The figure shows three views and two pictorial views of one solid part (mm, origin at its lowest corner). Answer the questions. Give positions to 0.01 mm unless a question says otherwise; leave off trailing zeros. Loops run counter-clockwise (first coordinate to the right, second up) from the corner with the lowest first, then second, coordinate; pieces in that order, holes last. Notation, with made-up numbers: (-20, 83.25) - (15, 83.25) arc R21 cw to (15, 119.25) - close; hole circle Ø1 at (-11, 35). An arc over 180 degrees is marked (long way). Use CSV: the item, a comma, the result in double quotes.
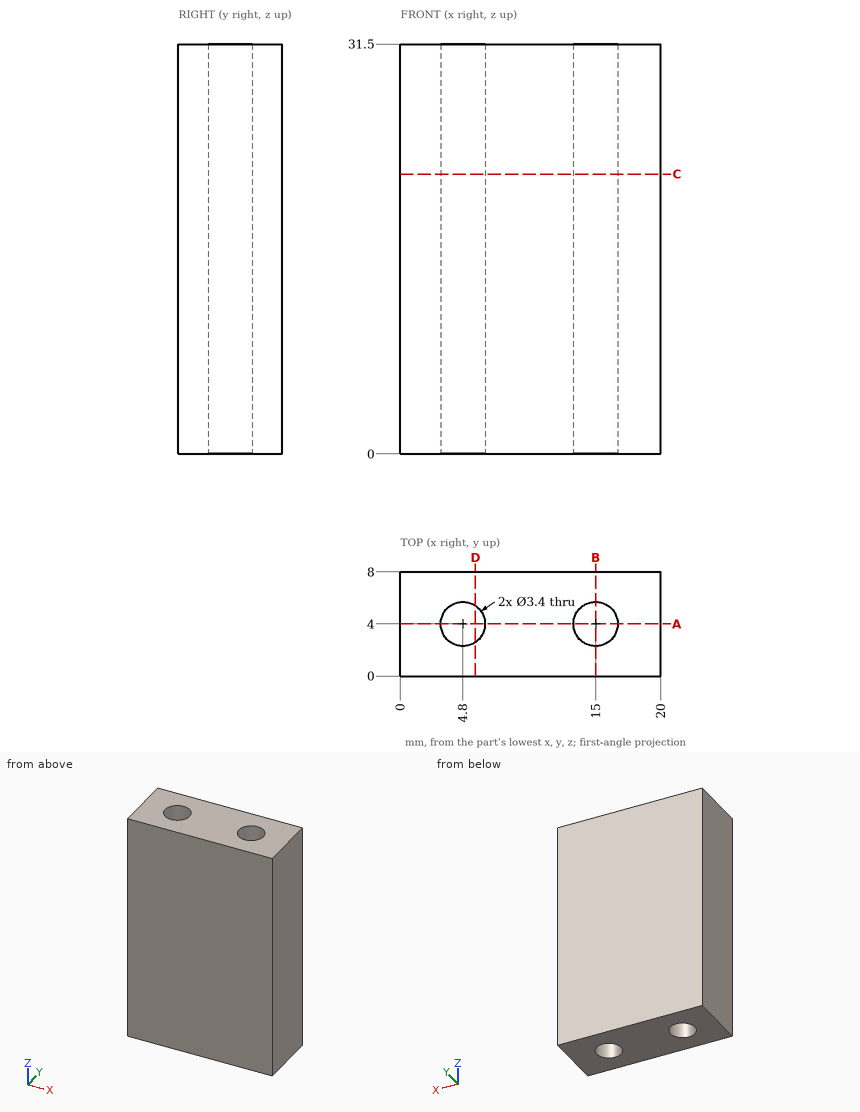
Item 1: Find the intervals of material crossed by line 1 (Y direction, x = 15, z = 6); line 2 (X direction, y = 4.25, z = 19); line 3 (Y direction, x = 16, z = 20.5), in increasing order.
Determined:
line 1,"y = 0 to 2.3, 5.7 to 8"
line 2,"x = 0 to 3.12, 6.48 to 13.32, 16.68 to 20"
line 3,"y = 0 to 2.63, 5.37 to 8"
Item 2: A cutting plane is placed at D-D on x = 5.75. Determine the outline of the cut face in (y, z).
Determined:
outline,"(0, 0) - (2.59, 0) - (2.59, 31.5) - (0, 31.5) - close; (5.41, 0) - (8, 0) - (8, 31.5) - (5.41, 31.5) - close"
Item 3: A cutting plane is placed at B-B on x = 15. Determine the outline of the cut face in (y, z), and give its area (3 significant figures).
Determined:
outline,"(0, 0) - (2.3, 0) - (2.3, 31.5) - (0, 31.5) - close; (5.7, 0) - (8, 0) - (8, 31.5) - (5.7, 31.5) - close"
area,"145 mm²"
Item 4: A cutting plane is placed at A-A on y = 4. Determine the outline of the cut face in (x, z).
Determined:
outline,"(0, 0) - (3.1, 0) - (3.1, 31.5) - (0, 31.5) - close; (6.5, 0) - (13.3, 0) - (13.3, 31.5) - (6.5, 31.5) - close; (16.7, 0) - (20, 0) - (20, 31.5) - (16.7, 31.5) - close"
Item 5: A cutting plane is placed at C-C on z = 21.5. Determine the outline of the cut face in (x, y), and give its area (3 significant figures).
Determined:
outline,"(0, 0) - (20, 0) - (20, 8) - (0, 8) - close; hole circle Ø3.4 at (4.8, 4); hole circle Ø3.4 at (15, 4)"
area,"142 mm²"
